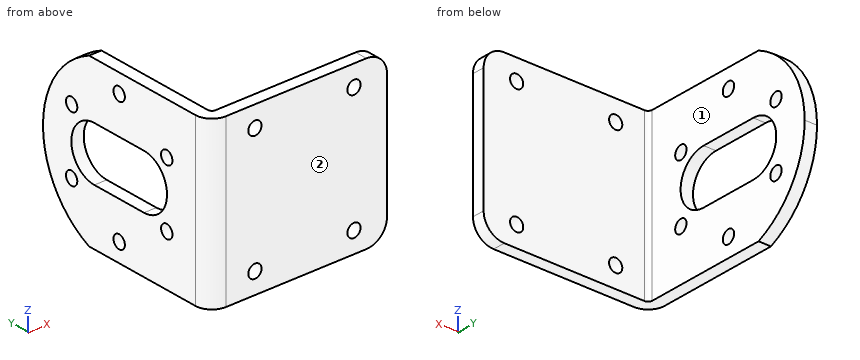
from build123d import *

# Parameters (mm, degrees)
SM_BASE_FLANGE_1_DEPTH      = 40
CUT_EXTRUDE_3_DEPTH         = 10
CUT_EXTRUDE_1_DEPTH         = 74.382559236
SKETCH_7_R                  = 1.6
CUT_EXTRUDE_2_DEPTH         = 74.382559236
SKETCH_9_R                  = 1.6
CUT_EXTRUDE_4_DEPTH         = 74.545904033
PATTERN_LINEAR_1_COUNT      = 2
PATTERN_LINEAR_1_PITCH      = 30
PATTERN_LINEAR_1_COUNT_DIR2 = 2
PATTERN_LINEAR_1_PITCH_DIR2 = 24
FILLET_1_R                  = 5


# Sheet-metal steps are written as plain solids
with BuildPart() as part:
    # Sketch 1 → 基材-凸緣1 (new body)
    with BuildSketch(Plane.XY):
        with BuildLine():
            Line((40, 0), (1, 0))
            ThreePointArc((1, 0), (0.292893219, 0.292893219), (0, 1))
            Line((0, 1), (0, 44))
            Line((0, 44), (-3, 44))
            Line((-3, 44), (-3, 1))
            ThreePointArc((-3, 1), (-1.828427125, -1.828427125), (1, -3))
            Line((1, -3), (40, -3))
            Line((40, -3), (40, 0))
        make_face()
    extrude(amount=SM_BASE_FLANGE_1_DEPTH)

    # 草圖8 → 除料-伸長3 (cut)
    with BuildSketch(Plane.ZY.offset(3)):
        with BuildLine():
            Line((0, 44), (0, 31.002788981))
            ThreePointArc((0, 31.002788981), (8.073899482, 40.465261916), (20, 44))
            Line((20, 44), (0, 44))
        make_face()
        with BuildLine():
            ThreePointArc((20, 44), (31.926100518, 40.465261916), (40, 31.002788981))
            Line((40, 31.002788981), (40, 44))
            Line((40, 44), (20, 44))
        make_face()
    extrude(amount=-CUT_EXTRUDE_3_DEPTH, mode=Mode.SUBTRACT)

    # 草圖6 → 除料-伸長1 (cut, through all)
    with BuildSketch(Plane.ZY.offset(3)):
        with BuildLine():
            Line((26.5, 29.5), (26.5, 15.5))
            ThreePointArc((26.5, 15.5), (20, 9), (13.5, 15.5))
            Line((13.5, 15.5), (13.5, 29.5))
            ThreePointArc((13.5, 29.5), (20, 36), (26.5, 29.5))
        make_face()
    extrude(amount=-CUT_EXTRUDE_1_DEPTH, mode=Mode.SUBTRACT)

    # 草圖7 → 除料-伸長2 (cut, through all)
    with BuildSketch(Plane.ZY.offset(3)):
        with Locations((4.5, 22.5)):
            Circle(SKETCH_7_R)
        with Locations((12.25, 9.076606241)):
            Circle(SKETCH_7_R)
        with Locations((27.75, 9.076606241)):
            Circle(SKETCH_7_R)
        with Locations((35.5, 22.5)):
            Circle(SKETCH_7_R)
        with Locations((27.75, 35.923393759)):
            Circle(SKETCH_7_R)
        with Locations((12.25, 35.923393759)):
            Circle(SKETCH_7_R)
    extrude(amount=-CUT_EXTRUDE_2_DEPTH, mode=Mode.SUBTRACT)

    # 草圖9 → 除料-伸長4 (cut, through all)
    with BuildSketch(Plane.XZ.offset(3)):
        with Locations(Location((32, 35, 0), (0, 0, 270))):
            Circle(SKETCH_9_R)
    cut_extrude_4 = extrude(amount=-CUT_EXTRUDE_4_DEPTH, mode=Mode.SUBTRACT)

    # 直線複製排列1: Cut-Extrude 4 2 × 2
    with Locations(*[(-j * PATTERN_LINEAR_1_PITCH_DIR2, 0, -i * PATTERN_LINEAR_1_PITCH) for i in range(PATTERN_LINEAR_1_COUNT) for j in range(PATTERN_LINEAR_1_COUNT_DIR2) if (i, j) != (0, 0)]):
        add(cut_extrude_4, mode=Mode.SUBTRACT)

    # 圓角1
    fillet_1_edges = [part.edges().sort_by_distance(p)[0] for p in [
        (40, -1.5, 40),
        (40, -1.5, 0),
    ]]
    fillet(fillet_1_edges, radius=FILLET_1_R)


solid = part.part
Geometry check sheet. Reference: the model listing, model coordinates, mm. Face numbers are marked on the shaded views. A direction names the side the tool comes from. Give positions to 0.01 mm unless a question says otherwise; leave off trailing zeros. Write each loop counter-clockwise with the first axis right and the second up, starting at its lowest first coordinate (ties: lowest second). Pieces come first, ordered by that corner, then holes. Notation, with made-up numbers: (18.5, -31) - (50.5, -31) arc R17 ccw to (50.5, -21) - close; hole circle Ø3 at (-29, 5). An arc over 180 degrees is marked (long way). Put each result on its own line as item: value.
1. Thickness scan on line 1 (Y direction, x = 36, z = 24); line 2 (X direction, y = -1, z = 5). Record the ranges inside material, lowest first.
Ans:
line 1: y = -3 to 0
line 2: x = -2.46 to 6.4, 9.6 to 30.4, 33.6 to 40
2. Sectioned sample at B-B, the plane z = 12.25. Enter the section's corners in (x, y).
Ans:
outline: (-3, 1) arc R4 ccw to (1, -3) - (40, -3) - (40, 0) - (1, 0) arc R1 cw to (0, 1) - (0, 7.48) - (-3, 7.48) - close; (-3, 10.68) - (0, 10.68) - (0, 34.32) - (-3, 34.32) - close; (-3, 37.52) - (0, 37.52) - (0, 42.58) - (-3, 42.58) - close
3. Go/stop test with flat-tipped pins: pin 1 (5 mm diameter, centred on y = 37.5, z = 32, fed in from +X); pin 2 (5 mm diameter, centred on x = 32, z = 5, fed in from +Y). Record where each tip stops, or that it passes through.
Ans:
pin 1: stops at x = 0
pin 2: stops at y = 0
4. Set-up check for the marked faces 1 and 2: record each of +Z, -Z, +X, -X, +Y, -Y from which the full face is reachable in a straight line by a thin tool's end or side.
Ans:
face 1: +Z, -Z, +X, +Y
face 2: +Z, -Z, +X, -X, -Y
5. Sectioned sample at D-D, the plane y = 4. Enter the section's corners in (x, z), plus the area to 3 significant figures.
Ans:
outline: (-3, 0) - (0, 0) - (0, 40) - (-3, 40) - close
area: 120 mm²
6. Sectioned sample at C-C, the plane z = 17. Enter the section's corners in (x, y).
Ans:
outline: (-3, 1) arc R4 ccw to (1, -3) - (40, -3) - (40, 0) - (1, 0) arc R1 cw to (0, 1) - (0, 9.73) - (-3, 9.73) - close; (-3, 35.27) - (0, 35.27) - (0, 43.79) - (-3, 43.79) - close
7. Sectioned sample at A-A, the plane y = 22.5. Enter the section's corners in (x, z), plus the area to 3 significant figures.
Ans:
outline: (-3, 0) - (0, 0) - (0, 2.9) - (-3, 2.9) - close; (-3, 6.1) - (0, 6.1) - (0, 13.5) - (-3, 13.5) - close; (-3, 26.5) - (0, 26.5) - (0, 33.9) - (-3, 33.9) - close; (-3, 37.1) - (0, 37.1) - (0, 40) - (-3, 40) - close
area: 61.8 mm²
